Design review of the part built by this model. Coordinates are the model's own, in mm. A direction names the side the tool comes from. Give positions to 0.01 mm unless a question says otherwise; leave off trailing zeros. Order: outer loops, then holes, each group sorted by start corner. A loop starts at its lowest first (then second) coordinate and runs counter-clockwise, first axis right, second up. Notation, with made-up numbers: (-17, -7.5) -> (20, -7.5) arc R18 cw to (20, 20.5) -> close; hole circle Ø11 at (21.25, -28). An arc over 180 degrees is marked (long way). One line per item, written item: value. Start each with the question number.
1) Consider section A-A (x = -8). State the section outline as (y, z) points, plus the area to 3 significant figures.
2) Consider section C-C (z = 21.5). State the section outline as (x, y) points.
3) Consider section D-D (z = -2). State the section outline as (x, y) points, plus the area to 3 significant figures.
4) For pin 1 (1 mm diameter, centred on y = -4, z = -0.5, fed in from -X); pin 2 (5.5 mm diameter, centred on x = -4.5, z = -2, fed in from -Y); pin 3 (2.5 mm diameter, centred on x = -0.5, y = -7, fed in from -Z), all flat-tipped, find the tip position at first contact; note any pin that passes through.
5) Tool access review of faces 1 (the face through (4, 7, 5)), 2 (the face through (2, -5, 20)), 3 (the face through (0, -5, -3)): name each direction out of +Z, -Z, +X, -X, +Y, -Y from which nothing blocks a thin tool from reaching the whole face with its end or side.
6) The part is to be moulded in two halves that separate along Z. For faces 4 (the face through (-1.08, -4.88, 11.23)), 5 (the face through (0, 0, 37)), 6 (the face through (-7.493, 0.33, 14.965)), 7 (the face through (2, -5, 17.5)), say which applies: released by +Z, released by -Z, zero draft, split by the parting line, or undercut.
7) Wall thickness on line 1 along Z through (x, y) = (2.5, -5.75); line 2 along Y through (x, z) = (1.25, 29.5); line 3 along X through (y, z) = (3.75, 13.5): over which ranges is each line inside the solid? List them lowest first. Write a range as from..to.
8) Consider section B-B (y = 7). State the section outline as (x, z) points, plus the area to 3 significant figures.
from build123d import *

# Parameters (mm, degrees)
SZKIC2_R                    = 10
DODANIE_WYCI_GNI_CIE1_DEPTH = 5
SZKIC3_R                    = 7.5
DODANIE_WYCI_GNI_CIE2_DEPTH = 5
SZKIC4_R                    = 5
DODANIE_WYCI_GNI_CIE3_DEPTH = 2.5
SZKIC5_R                    = 7.5
DODANIE_WYCI_GNI_CIE4_DEPTH = 5
SZKIC6_R                    = 5
DODANIE_WYCI_GNI_CIE5_DEPTH = 2.5
SZKIC7_R                    = 7.5
DODANIE_WYCI_GNI_CIE6_DEPTH = 5
SZKIC8_R                    = 6.5
DODANIE_WYCI_GNI_CIE7_DEPTH = 12
SZKIC10_W                   = 8
SZKIC10_H                   = 2
WYTNIJ_WYCI_GNI_CIE1_DEPTH  = 11
DODANIE_WYCI_GNI_CIE8_START = 5
SZKIC11_R                   = 10
DODANIE_WYCI_GNI_CIE8_DEPTH = 5
WYTNIJ_WYCI_GNI_CIE2_DEPTH  = 5


with BuildPart() as part:
    # Szkic2 → Dodanie-wyciągnięcie1 (new body)
    with BuildSketch(Plane.XY):
        Circle(SZKIC2_R)
    extrude(amount=DODANIE_WYCI_GNI_CIE1_DEPTH)

    # Szkic3 → Dodanie-wyciągnięcie2 (add)
    with BuildSketch(Plane.XY.offset(5)):
        Circle(SZKIC3_R)
    extrude(amount=DODANIE_WYCI_GNI_CIE2_DEPTH)

    # Szkic4 → Dodanie-wyciągnięcie3 (add)
    with BuildSketch(Plane.XY.offset(10)):
        Circle(SZKIC4_R)
    extrude(amount=DODANIE_WYCI_GNI_CIE3_DEPTH)

    # Szkic5 → Dodanie-wyciągnięcie4 (add)
    with BuildSketch(Plane.XY.offset(12.5)):
        Circle(SZKIC5_R)
    extrude(amount=DODANIE_WYCI_GNI_CIE4_DEPTH)

    # Szkic6 → Dodanie-wyciągnięcie5 (add)
    with BuildSketch(Plane.XY.offset(17.5)):
        Circle(SZKIC6_R)
    extrude(amount=DODANIE_WYCI_GNI_CIE5_DEPTH)

    # Szkic7 → Dodanie-wyciągnięcie6 (add)
    with BuildSketch(Plane.XY.offset(20)):
        Circle(SZKIC7_R)
    extrude(amount=DODANIE_WYCI_GNI_CIE6_DEPTH)

    # Szkic8 → Dodanie-wyciągnięcie7 (add)
    with BuildSketch(Plane.XY.offset(25)):
        Circle(SZKIC8_R)
    extrude(amount=DODANIE_WYCI_GNI_CIE7_DEPTH)

    # Szkic10 → Wytnij-wyciągnięcie1 (cut)
    with BuildSketch(Plane.XY.offset(37)):
        with Locations((0, 6.5)):
            Rectangle(SZKIC10_W, SZKIC10_H)
        with Locations((0, -6.5)):
            Rectangle(SZKIC10_W, SZKIC10_H)
    extrude(amount=-WYTNIJ_WYCI_GNI_CIE1_DEPTH, mode=Mode.SUBTRACT)

    # Szkic11 → Dodanie-wyciągnięcie8 (add)
    with BuildSketch(Plane(origin=(0, 0, 0), x_dir=(-1, 0, 0), z_dir=(0, 0, -1)).offset(DODANIE_WYCI_GNI_CIE8_START)):
        Circle(SZKIC11_R)
    extrude(amount=-DODANIE_WYCI_GNI_CIE8_DEPTH)

    # Szkic13 → Wytnij-wyciągnięcie2 (cut)
    with BuildSketch(Plane(origin=(0, 0, -5), x_dir=(-1, 0, 0), z_dir=(0, 0, -1))):
        with BuildLine():
            Line((-8.660254038, -5), (8.660254038, -5))
            ThreePointArc((8.660254038, -5), (0, -10), (-8.660254038, -5))
        make_face()
        with BuildLine():
            Line((-8.660254038, 5), (8.660254038, 5))
            ThreePointArc((8.660254038, 5), (0, 10), (-8.660254038, 5))
        make_face()
    extrude(amount=-WYTNIJ_WYCI_GNI_CIE2_DEPTH, mode=Mode.SUBTRACT)

    # Sfazowanie1: read off the stored shape, not the designer's step
    # Sfazowanie1 outline → Sfazowanie1 (revolve, cut)
    with BuildSketch(Plane.XZ):
        Polygon((6.5, 37.000001298), (5.499998702, 37.000001298), (6.5, 36), align=None)
    revolve(axis=Axis((0, 0, 0), (0, 0, 1)), mode=Mode.SUBTRACT)


solid = part.part
Checked values:
1. outline: (-6, 0) -> (-5, 0) -> (-5, -5) -> (5, -5) -> (5, 0) -> (6, 0) -> (6, 5) -> (-6, 5) -> close
1. area: 110 mm^2
2. outline: circle Ø15 at (0, 0)
3. outline: (-8.66, -5) -> (8.66, -5) arc R10 ccw to (8.66, 5) -> (-8.66, 5) arc R10 ccw to start
3. area: 191 mm^2
4. pin 1: stops at x = -9.37
4. pin 2: stops at y = -9.65
4. pin 3: stops at z = 0
5. face 1: +Z
5. face 2: none
5. face 3: -Z, +X, -X, -Y
6. face 4: undercut
6. face 5: released by +Z
6. face 6: zero draft
6. face 7: undercut
7. line 1: z = 0..10, 12.5..17.5, 20..26
7. line 2: y = -5.5..5.5
7. line 3: x = -6.5..6.5
8. outline: (-7.14, 0) -> (7.14, 0) -> (7.14, 5) -> (2.69, 5) -> (2.69, 10) -> (-2.69, 10) -> (-2.69, 5) -> (-7.14, 5) -> close; (-2.69, 12.5) -> (2.69, 12.5) -> (2.69, 17.5) -> (-2.69, 17.5) -> close; (-2.69, 20) -> (2.69, 20) -> (2.69, 25) -> (-2.69, 25) -> close
8. area: 152 mm^2
